from build123d import *

# Parameters (mm, degrees)
F1_DEPTH = 25.4
F2_DEPTH = 25.4


with BuildPart() as f1:
    # F0 (on Top) → F1 (new body)
    with BuildSketch(Plane.XY):
        Polygon((-34.6818976104, 30.9372004122), (-56.627497077, 30.9372004122), (-56.627497077, -40.0811992586), (0, -40.0811992586), (56.627497077, -40.0811992586), (56.627497077, 30.9372004122), (34.6818976104, 30.9372004122), (34.6818976104, 61.1124001443), (0, 61.1124001443), (-34.6818976104, 61.1124001443), align=None)
        with BuildLine():
            ThreePointArc((0, -32.6451188582), (-32.6451188582, 0), (0, 32.6451188582))
            ThreePointArc((0, 32.6451188582), (32.6451188582, 0), (0, -32.6451188582))
        make_face(mode=Mode.SUBTRACT)
    extrude(amount=F1_DEPTH)

    # F0 (on Top) → F2 (join)
    with BuildSketch(Plane.XY):
        Polygon((-34.6818976104, 30.9372004122), (-56.627497077, 30.9372004122), (-56.627497077, -40.0811992586), (0, -40.0811992586), (56.627497077, -40.0811992586), (56.627497077, 30.9372004122), (34.6818976104, 30.9372004122), (34.6818976104, 61.1124001443), (0, 61.1124001443), (-34.6818976104, 61.1124001443), align=None)
        with BuildLine():
            ThreePointArc((0, -32.6451188582), (-32.6451188582, 0), (0, 32.6451188582))
            ThreePointArc((0, 32.6451188582), (32.6451188582, 0), (0, -32.6451188582))
        make_face(mode=Mode.SUBTRACT)
    extrude(amount=F2_DEPTH)


solid = f1.part
Can you work these out from the model? Positions are in its coordinate system, mm. A direction names the side the tool comes from. Give positions to 0.01 mm unless a question says otherwise; leave off trailing zeros. Loops run counter-clockwise (first coordinate to the right, second up) from the corner with the lowest first, then second, coordinate; pieces in that order, holes last. Notation, with made-up numbers: (72, 79) - (85, 79) arc R31 cw to (85, 115) - close; hole circle Ø7 at (11, 36). An arc over 180 degrees is marked (long way). One line per item, written item: value.
(1) If we section it at A-A, the plane y = 0: List the corners of the cut face in (x, z) for me, plus the area to 3 significant figures.
Verdict:
outline: (-56.63, 0) - (-32.65, 0) - (-32.65, 25.4) - (-56.63, 25.4) - close; (32.65, 0) - (56.63, 0) - (56.63, 25.4) - (32.65, 25.4) - close
area: 1,220 mm^2
(2) If we section it at C-C, the plane z = 4.5: List the corners of the cut face in (x, y) for me.
Verdict:
outline: (-56.63, -40.08) - (56.63, -40.08) - (56.63, 30.94) - (34.68, 30.94) - (34.68, 61.11) - (-34.68, 61.11) - (-34.68, 30.94) - (-56.63, 30.94) - close; hole circle Ø65.29 at (0, 0)
(3) If we section it at B-B, the plane x = 0: List the corners of the cut face in (y, z) for me, plus the area to 3 significant figures.
Verdict:
outline: (-40.08, 0) - (-32.65, 0) - (-32.65, 25.4) - (-40.08, 25.4) - close; (32.65, 0) - (61.11, 0) - (61.11, 25.4) - (32.65, 25.4) - close
area: 912 mm^2
(4) On a 3-axis mill with a long thin cutter (end or side, diameter ignored), from which of +Z, -Z, +X, -X, +Y, -Y can I reach the whole of each face in a straight line? I mean faces 4 (the face through (46, 30.937, 13)), 5 (the face through (-46, 30.937, 13)), 6 (the face through (0, 61.112, 13)). Say none if no direction works.
Verdict:
face 4: +Z, -Z, +X, +Y
face 5: +Z, -Z, -X, +Y
face 6: +Z, -Z, +X, -X, +Y
(5) I need wall thicknesses on line 1 along X through (y, z) = (0, 6.25); line 2 along Y through (x, z) = (8.5, 2); line 3 along X through (y, z) = (-23, 17.5). Which ranges of each line are inside material? Lowest first, please.
Verdict:
line 1: -56.63 to -32.65, 32.65 to 56.63
line 2: -40.08 to -31.52, 31.52 to 61.11
line 3: -56.63 to -23.17, 23.17 to 56.63
(6) I'm going to push flat-ended pins straight in: pin 1 (7.5 mm diameter, centred on y = 49, z = 12, fed in from -X); pin 2 (11 mm diameter, centred on x = 47.5, z = 15, fed in from +Y); pin 3 (7.5 mm diameter, centred on y = 51, z = 8, fed in from +X). Where does each tip first touch, or does it pass through?
Verdict:
pin 1: x = -34.68
pin 2: y = 30.94
pin 3: x = 34.68
(7) If we mould it in two halves opening along Y, with no side actions, what happens to faces 1 (the face through (-12.503, 30.156, 12.522)), 2 (the face through (-1, -40.081, 13)), 3 (the face through (-1, 34, 25.4))? For each: released by +Y, released by -Y, zero draft, split by the parting line, or undercut.
Verdict:
face 1: undercut
face 2: released by -Y
face 3: zero draft
(8) If we section it at D-D, the plane y = 37.5: List the corners of the cut face in (x, z) for me, plus the area to 3 significant figures.
Verdict:
outline: (-34.68, 0) - (34.68, 0) - (34.68, 25.4) - (-34.68, 25.4) - close
area: 1,760 mm^2
